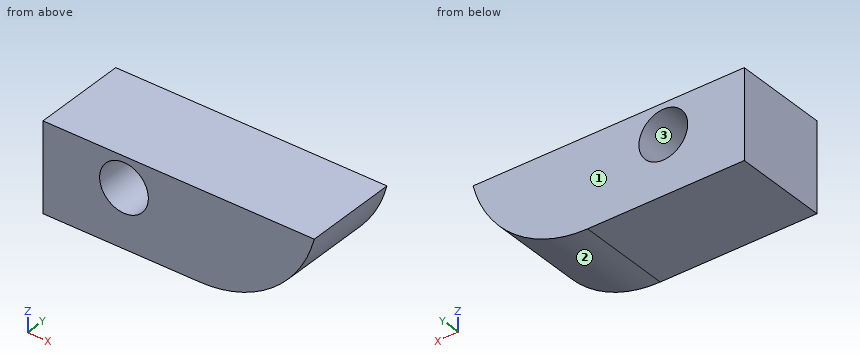
```python
from build123d import *

# Parameters (mm, degrees)
F0_W        = 73.1619596481
F0_H        = 24.0233289078
F0_R        = 6.5745281788
F1_DEPTH    = 25.4
F2_T1_DEPTH = 179.9105347495


# Not quite as in the source:
# - a fillet or chamfer that OpenCascade refuses, or shapes differently, is made with other operations: its cross-section is extruded or revolved along the edge and cut away or added


with BuildPart() as f1:
    # F0 (on Front) → F1 (new body)
    with BuildSketch(Plane.XZ):
        with Locations((-0.2729967237, -3.8218903355)):
            Rectangle(F0_W, F0_H)
        with Locations((-15.0145851076, 0)):
            Circle(F0_R, mode=Mode.SUBTRACT)
    extrude(amount=F1_DEPTH)

    # F2: fillet of radius 31.8869327318 on 1 edges, made by hand

    # F2_s2 → F2_t1 (cut)
    with BuildSketch(Plane.XZ.offset(-77.2552673747)):
        with BuildLine():
            ThreePointArc((5.4058761505, -15.8335547894), (24.9766486554, -9.1212390876), (36.3079831004, 8.1897741184))
            Line((36.3079831004, 8.1897741184), (36.3079831004, -15.8335547894))
            Line((36.3079831004, -15.8335547894), (5.4058761505, -15.8335547894))
        make_face()
    extrude(amount=F2_T1_DEPTH, mode=Mode.SUBTRACT)


solid = f1.part
```
CAD build for the part. Positions are in the model's coordinates, mm. Face numbers are marked on the shaded views. Coordinates: 2 decimals unless noted, no trailing zeros. Order: outer loops, then holes, each group sorted by start corner. A loop starts at its lowest first (then second) coordinate and runs counter-clockwise, first axis right, second up.
(1) Saw through at B-B, the plane y = -5. Write the cut outline in (x, z), and give its area (3 significant figures).
Solution:
outline: (-36.85, -15.83) - (5.41, -15.83) arc R31.89 ccw to (36.31, 8.19) - (-36.85, 8.19) - close; hole circle Ø13.15 at (-15.01, 0)
area: 1,430 mm2
(2) Pin check, flat tips, straight feed: pin 1 Ø2 at (y, z) = (-20, -11) entering from +X; pin 2 Ø4 at (x, y) = (27.5, -20) entering from -Z; pin 3 Ø1 at (y, z) = (-6, -0.5) entering from +X. Stop position of each tip, or through.
Solution:
pin 1: stops at x = 23.79
pin 2: stops at z = -8.71
pin 3: stops at x = 32.96
(3) Mould opens along X. For the marked faces 1, 2 and 3 say: released by +X, released by -X, zero draft, split by the parting line, or undercut.
Solution:
face 1: zero draft
face 2: released by +X
face 3: undercut
(4) Saw through at A-A, the plane z = -3. Write the cut outline in (x, y), and give its area (3 significant figures).
Solution:
outline: (-36.85, -25.4) - (-20.86, -25.4) - (-20.86, 0) - (-36.85, 0) - close; (-9.16, -25.4) - (30.97, -25.4) - (30.97, 0) - (-9.16, 0) - close
area: 1,430 mm2
(5) Saw through at C-C, the plane z = 0. Write the cut outline in (x, y).
Solution:
outline: (-36.85, -25.4) - (-21.59, -25.4) - (-21.59, 0) - (-36.85, 0) - close; (-8.44, -25.4) - (32.96, -25.4) - (32.96, 0) - (-8.44, 0) - close
(6) Saw through at D-D, the plane x = 29. Write the cut outline in (y, z).
Solution:
outline: (-25.4, -5.4) - (0, -5.4) - (0, 8.19) - (-25.4, 8.19) - close
(7) Drill centre lines: L1, parallel to X at y = -3, z = -4.25; L2, parallel to X at y = -20.5, z = -5.5; L3, parallel to Z at x = -13.5, y = -23. Where is each one in solid material? Low to high.
Solution:
L1: x = -36.85 to -20.03, -10 to 29.99
L2: x = -36.85 to -18.62, -11.41 to 28.91
L3: z = -15.83 to -6.4, 6.4 to 8.19
